```python
from build123d import *

# Parameters (mm, degrees)
ESQUISSE1_R        = 1
BOSS_EXTRU_2_DEPTH = 1.5
ESQUISSE2_R        = 10
BOSS_EXTRU_3_DEPTH = 15


with BuildPart() as part:
    # Esquisse1 → Boss.-Extru.2 (new body)
    with BuildSketch(Plane.XY):
        with BuildLine():
            Line((20.277172368, -9.884393064), (20.277172368, -1.384393064))
            ThreePointArc((20.277172368, -1.384393064), (21.777172368, 0.115606936), (20.277172368, 1.615606936))
            Line((20.277172368, 1.615606936), (20.277172368, 10.115606936))
            Line((20.277172368, 10.115606936), (-19.722827632, 10.115606936))
            Line((-19.722827632, 10.115606936), (-19.722827632, -9.884393064))
            Line((-19.722827632, -9.884393064), (20.277172368, -9.884393064))
        make_face()
        with Locations((20.277172368, 0.115606936)):
            Circle(ESQUISSE1_R, mode=Mode.SUBTRACT)
    extrude(amount=BOSS_EXTRU_2_DEPTH)

    # Esquisse2 → Boss.-Extru.3 (add)
    with BuildSketch(Plane.XY):
        with Locations((8.277172368, 0.047190926)):
            Circle(ESQUISSE2_R)
    extrude(amount=-BOSS_EXTRU_3_DEPTH)


solid = part.part
```
Work out the finished part from the listing and answer in its coordinate system (mm). A direction names the side the tool comes from. Round coordinates to 2 decimals unless told otherwise and drop trailing zeros. Write each loop counter-clockwise with the first axis right and the second up, starting at its lowest first coordinate (ties: lowest second). Pieces come first, ordered by that corner, then holes.
1) A cutting plane is placed at B-B on x = 17. Determine the outline of the cut face in (y, z), and give its area (3 significant figures).
2) Flat-ended cylindrical pins translate along their axes: P1, Ø1.5, axis at x = 15.5, z = -9, coming from the +Y side; P2, Ø0.8, axis at y = 6, z = 0.5, coming from the +X side; P3, Ø4, axis at x = 12, z = -7, coming from the -Y side. Find the tip coordinate at first contact, or state that the pin passes through.
3) A cutting plane is placed at A-A on y = -3.25. Determine the outline of the cut face in (x, z), and give its area (3 significant figures).
4) Consider probe 1 along Y at (x, z) = (8.5, -5.75); probe 2 along Z at (x, y) = (-2.5, -8.25); probe 3 along X at (y, z) = (1.75, -11.75). Determine where each line is inside the solid, lowest interval first.
5) Which of the six approach directions +Z, -Z, +X, -X, +Y, -Y give full straight-line access (tool end or side, diameter ignored) to faces 4 (the face through (8, 0, -15)), 5 (the face through (20.277, -6, 1)), 6 (the face through (17.8, 3.1, -7.4)), 7 (the face through (20.277, 6, 1))?
6) A cutting plane is placed at C-C on z = -12.75. Determine the outline of the cut face in (x, y), and give its area (3 significant figures).
7) Determine the mould class of faces 1 (the face through (21.777, 0.083, 0.74)), 2 (the face through (19.28, 0.16, 0.74)), 3 (the face through (0, -9.884, 1)) for opening direction X: pulls with the +X half, pulls with the -X half, needs draft (parallel to the pull), parting line crosses it, or undercut.
8) A cutting plane is placed at D-D on x = -9. Determine the outline of the cut face in (y, z).
Entries:
1. outline: (-9.88, 0) - (-4.84, 0) - (-4.84, -15) - (4.94, -15) - (4.94, 0) - (10.12, 0) - (10.12, 1.5) - (-9.88, 1.5) - close
1. area: 177 mm2
2. P1: stops at y = 7.67
2. P2: stops at x = 20.28
2. P3: stops at y = -9.8
3. outline: (-19.72, 0) - (-1.16, 0) - (-1.16, -15) - (17.72, -15) - (17.72, 0) - (20.28, 0) - (20.28, 1.5) - (-19.72, 1.5) - close
3. area: 343 mm2
4. probe 1: y = -9.95 to 10.04
4. probe 2: z = 0 to 1.5
4. probe 3: x = -1.58 to 18.13
5. face 4: -Z, +X, -X, +Y, -Y
5. face 5: +Z, -Z, +X, -Y
5. face 6: -Z
5. face 7: +Z, -Z, +X, +Y
6. outline: circle Ø20 at (8.28, 0.05)
6. area: 314 mm2
7. face 1: pulls with the +X half
7. face 2: undercut
7. face 3: needs draft
8. outline: (-9.88, 0) - (10.12, 0) - (10.12, 1.5) - (-9.88, 1.5) - close
